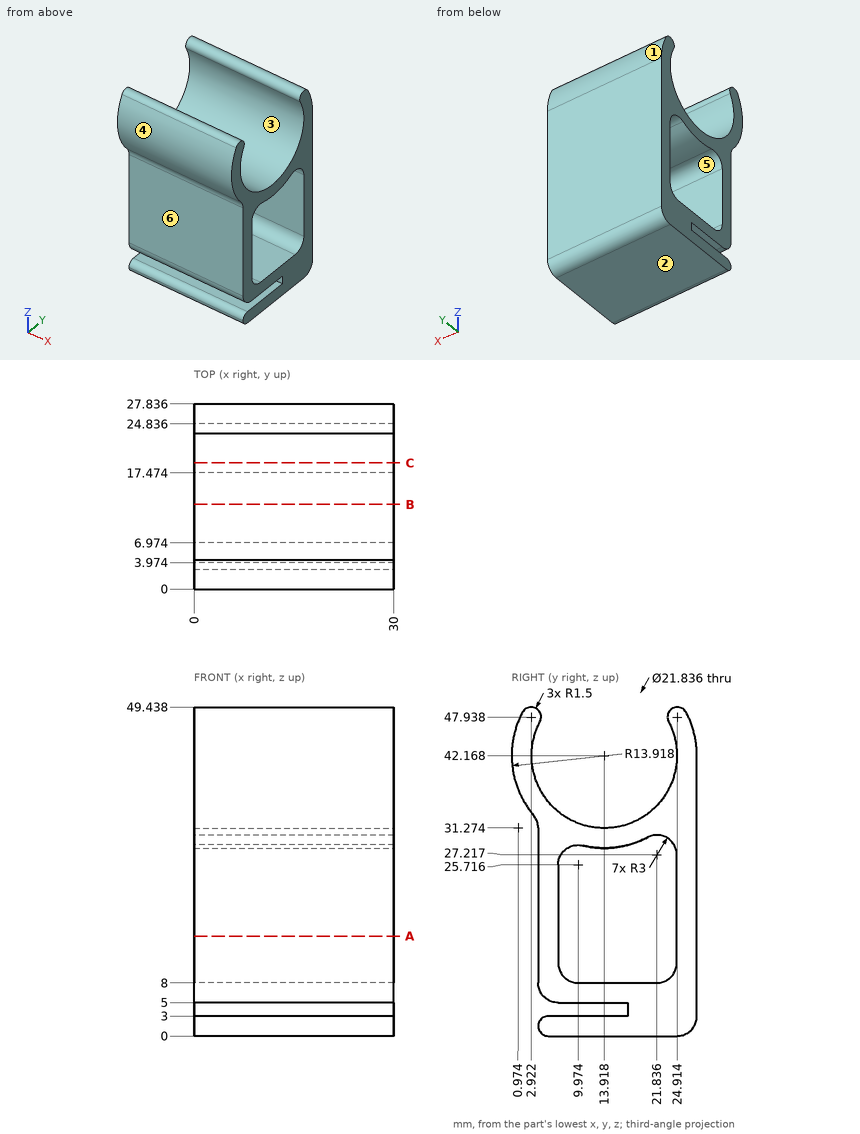
Source: three-view drawing plus pictorial views. Frame: mm from the lowest corner of the part. A direction names the side the tool comes from. Round coordinates to 2 decimals unless told otherwise and drop trailing zeros. Write each loop counter-clockwise with the first axis right and the second up, starting at its lowest first coordinate (ties: lowest second). Pieces come first, ordered by that corner, then holes. Notation, with made-up numbers: M -9.5,20 L 13.5,20 A20 ccw 13.5,46 Z; hole C -33,-32.75 d1. An arc over 180 degrees is marked long. Write each question's results on one line, items separated by ' | '.
Q1. Draft query along Y for the marked faces 1, 2 and 3. Return one class per face: released by +Y, released by -Y, zero draft, split by the parting line, or undercut.
Results:
face 1: released by +Y | face 2: zero draft | face 3: undercut
Q2. Pin query (flat end, axial travel): P1, Ø1, axis at x = 20, y = 19, coming from the +Z side (1 decimal); P2, Ø8, axis at x = 22, z = 17, coming from the -Y side; P3, Ø6, axis at x = 17.5, y = 15.5, coming from the +Z side; P4, Ø3, axis at x = 5.5, y = 5, coming from the -Z side. Return the tip coordinate at first contact, or that it passes through.
Results:
P1: stops at z = 32.8 | P2: stops at y = 3.97 | P3: stops at z = 32.26 | P4: stops at z = 0
Q3. Section query C-C (y = 19). Return loops of the section in (x, z) (1 decimal).
Results:
outline: M 0,0 L 30,0 L 30,8 L 0,8 Z; M 0,29.2 L 30,29.2 L 30,32.5 L 0,32.5 Z
Q4. Section query B-B (y = 12.75). Return loops of the section in (x, z).
Results:
outline: M 0,0 L 30,0 L 30,3 L 0,3 Z; M 0,5 L 30,5 L 30,8 L 0,8 Z; M 0,28.3 L 30,28.3 L 30,31.31 L 0,31.31 Z
Q5. Access query for the marked faces 4, 5 and 6. Directions: +Z, -Z, +X, -X, +Y, -Y. A direction counts if a zero-diameter tool reaches every point of the face in a straight line with its end or side. Return the directions, or none.
Results:
face 4: +X, -X, -Y | face 5: +X, -X | face 6: -Z, +X, -X, -Y
Q6. Line query: line 1 along Z through (x, y) = (23, 13.5); line 2 along Y through (x, z) = (11, 16); line 3 along Z through (x, y) = (6.5, 24) (1 decimal). Output: solid intervals per line, ascending.
Results:
line 1: z = 0 to 3, 5 to 8, 28.26 to 31.26 | line 2: y = 3.97 to 6.97, 24.84 to 27.84 | line 3: z = 0 to 8.9, 29.3 to 38, 46.4 to 49.1
Q7. Section query A-A (z = 15). Return loops of the section in (x, y), and give its area (3 significant figures).
Results:
outline: M 0,3.97 L 30,3.97 L 30,6.97 L 0,6.97 Z; M 0,24.84 L 30,24.84 L 30,27.84 L 0,27.84 Z | area: 180 mm^2
